Part model, mm, in its own coordinate system. Face numbers are marked on the shaded views. A direction names the side the tool comes from. Coordinates: 2 decimals unless noted, no trailing zeros. Loops run counter-clockwise (first coordinate to the right, second up) from the corner with the lowest first, then second, coordinate; pieces in that order, holes last. Notation, with made-up numbers: (18.25, 87) - (45.25, 87) arc R32 ccw to (45.25, 117) - close; hole circle Ø2 at (15, -26.75). An arc over 180 degrees is marked (long way). Use a Markdown table: item, result. Add a question column.
1. Pull direction Y, two halves, no side cores. Call the marked faces 1, 2 and 3: pulls with the +Y half, pulls with the -Y half, needs draft (parallel to the pull), parting line crosses it, or undercut.
2. Wall check: probe 1 along Z at (x, y) = (8, 0.1); probe 2 along Z at (x, y) = (1.25, 0.1); probe 3 along Y at (x, z) = (8, 0.5). Give the ranges that are in metal, low to high. Write a range as [from, to].
3. Drop flat-ended pins along their axis: pin 1 (2 mm diameter, centred on x = 17.5, y = -1.5, fed in from -Z); pin 2 (1 mm diameter, centred on x = 4, z = 1.5, fed in from +Y). Give the stop position or say it passes through.
4. 3-axis set-ups, long thin cutter, end or side, ignore diameter. For the marked faces 4 and 5: which of +Z, -Z, +X, -X, +Y, -Y reach the whole face in a straight line?
5. Band-saw the part on A-A, the plane x = 10. Give the cut face in (y, z).
from build123d import *

# Parameters (mm, degrees)
HEXAGONSOCKET_DEPTH = 2


with BuildPart() as part:
    # Sketch1 → Base (revolve)
    with BuildSketch(Plane.XY):
        Polygon((0, 0), (20, 0), (20, 1.75), (19.25, 2.5), (0.433, 2.5), (0, 2.067), align=None)
    revolve(axis=Axis((-10.745014543, 0, 0), (1, 0, 0)))

    # Sketch2 → HexagonSocket (cut)
    with BuildSketch(Plane(origin=(0, -0.021932325, 0.010138848), x_dir=(0, 0, 1), z_dir=(-1, 0, 0))):
        Polygon((1.433236825, 0.021932325), (0.711548988, 1.271932325), (-0.731826685, 1.271932325), (-1.453514521, 0.021932325), (-0.731826685, -1.228067675), (0.711548988, -1.228067675), align=None)
    extrude(amount=-HEXAGONSOCKET_DEPTH, mode=Mode.SUBTRACT)

    # Sketch3 → Cut-Revolve1 (revolve, cut)
    with BuildSketch(Plane.XY):
        Polygon((2, 1.25), (2.721687837, 0), (2, 0), align=None)
    revolve(axis=Axis((-3.144113667, 0, 0), (1, 0, 0)), mode=Mode.SUBTRACT)


solid = part.part
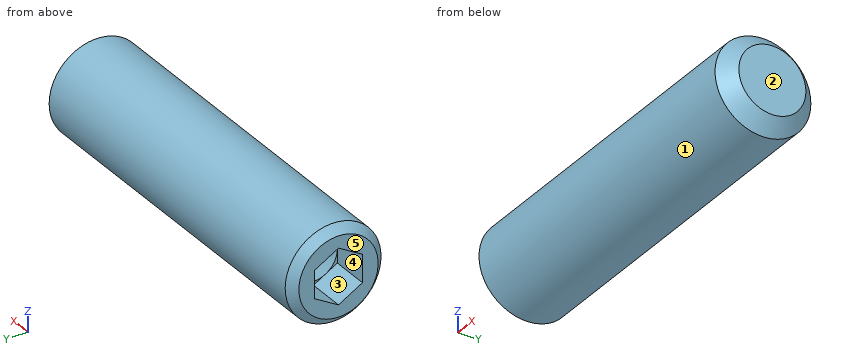
Geometry check:
| question | item | result |
|---|---|---|
| 1 | face 1 | parting line crosses it |
| 1 | face 2 | needs draft |
| 1 | face 3 | undercut |
| 2 | probe 1 | z = [-2.5, 2.5] |
| 2 | probe 2 | z = [-2.5, -1.39], [1.39, 2.5] |
| 2 | probe 3 | y = [-2.45, 2.45] |
| 3 | pin 1 | stops at z = -2.45 |
| 3 | pin 2 | stops at y = 2.29 |
| 4 | face 4 | -X |
| 4 | face 5 | +Z, -Z, -X, +Y, -Y |
| 5 | outline | circle Ø5 at (0, 0) |
